```python
from build123d import *

# Parameters (mm, degrees)
SKETCH_1_W      = 9.8
SKETCH_1_H      = 0.68
EXTRUDE_1_DEPTH = 9.8
EXTRUDE_2_DEPTH = 0.46


with BuildPart() as part:
    # Эскиз1 → Бобышка-Вытянуть1 (new body)
    with BuildSketch(Plane(origin=(0, 0, 0), x_dir=(0, 0, -1), z_dir=(1, 0, 0))):
        with Locations((-2.397426888, 0.51364793)):
            Rectangle(SKETCH_1_W, SKETCH_1_H)
    extrude(amount=EXTRUDE_1_DEPTH)

    # Эскиз3 → Бобышка-Вытянуть2 (add)
    with BuildSketch(Plane(origin=(0, 0.85364793, 0), x_dir=(1, 0, 0), z_dir=(0, 1, 0))):
        Polygon((7.63, 2.352573112), (2.17, 2.352573112), (0.15, 0.332573112), (0.15, -5.127426888), (2.17, -7.147426888), (7.63, -7.147426888), (9.65, -5.127426888), (9.65, 0.332573112), align=None)
    extrude(amount=EXTRUDE_2_DEPTH)


solid = part.part
```
Here's how the part is built. I have some questions about the finished solid (model axes, mm). A direction names the side the tool comes from. Give positions to 0.01 mm unless a question says otherwise; leave off trailing zeros. Loops run counter-clockwise (first coordinate to the right, second up) from the corner with the lowest first, then second, coordinate; pieces in that order, holes last. Notation, with made-up numbers: M -30,73.5 L -14,73.5 A30 cw -14,97.5 Z; hole C 28.5,51 d7. An arc over 180 degrees is marked long. Return JSON: item names as keys, results as strings.
Item 1: Imagine slicing it at A-A on y = 1.1. List the corners of the cut face in (x, z) for me, then the cut area to 3 significant figures.
A:
{"outline": "M 0.15,-0.33 L 2.17,-2.35 L 7.63,-2.35 L 9.65,-0.33 L 9.65,5.13 L 7.63,7.15 L 2.17,7.15 L 0.15,5.13 Z", "area": "82.1 mm^2"}
Item 2: Please list where these lines run through material, in increasing order: line 1 (X direction, y = 0.95, z = 4.75); line 2 (Z direction, x = 5.5, y = 0.95); line 3 (Z direction, x = 1.25, y = 1.15).
A:
{"line 1": "x = 0.15 to 9.65", "line 2": "z = -2.35 to 7.15", "line 3": "z = -1.43 to 6.23"}
Item 3: Thinking about a two-plate mould opening in Z: for faces 1 (the flat face through (5, 0.174, 2)), 2 (the flat face through (1.146, 1.08, 6.123)), 3 (the flat face through (1.174, 1.08, -1.357)), which applies, released by +Z, released by -Z, zero draft, split by the parting line, or undercut?
A:
{"face 1": "zero draft", "face 2": "released by +Z", "face 3": "released by -Z"}
Item 4: On a 3-axis mill with a long thin cutter (end or side, diameter ignored), from which of +Z, -Z, +X, -X, +Y, -Y can I reach the whole of each face in a straight line? I mean faces 4 (the flat face through (8.65, 1.08, -1.33)), 5 (the flat face through (8.63, 1.08, 6.15)), 6 (the flat face through (9, 0.854, 6)). Say none if no direction works.
A:
{"face 4": "-Z, +X, +Y", "face 5": "+Z, +X, +Y", "face 6": "+Y"}
Item 5: Imagine slicing it at B-B on x = 8. List the corners of the cut face in (y, z) for me.
A:
{"outline": "M 0.17,-2.5 L 0.85,-2.5 L 0.85,-1.98 L 1.31,-1.98 L 1.31,6.78 L 0.85,6.78 L 0.85,7.3 L 0.17,7.3 Z"}
